Could you check a few things on this drawing? It's one solid part, dimensions in mm from its lowest x, y, z. A direction names the side the tool comes from. Give positions to 0.01 mm unless a question says otherwise; leave off trailing zeros. Order: outer loops, then holes, each group sorted by start corner. A loop starts at its lowest first (then second) coordinate and runs counter-clockwise, first axis right, second up.
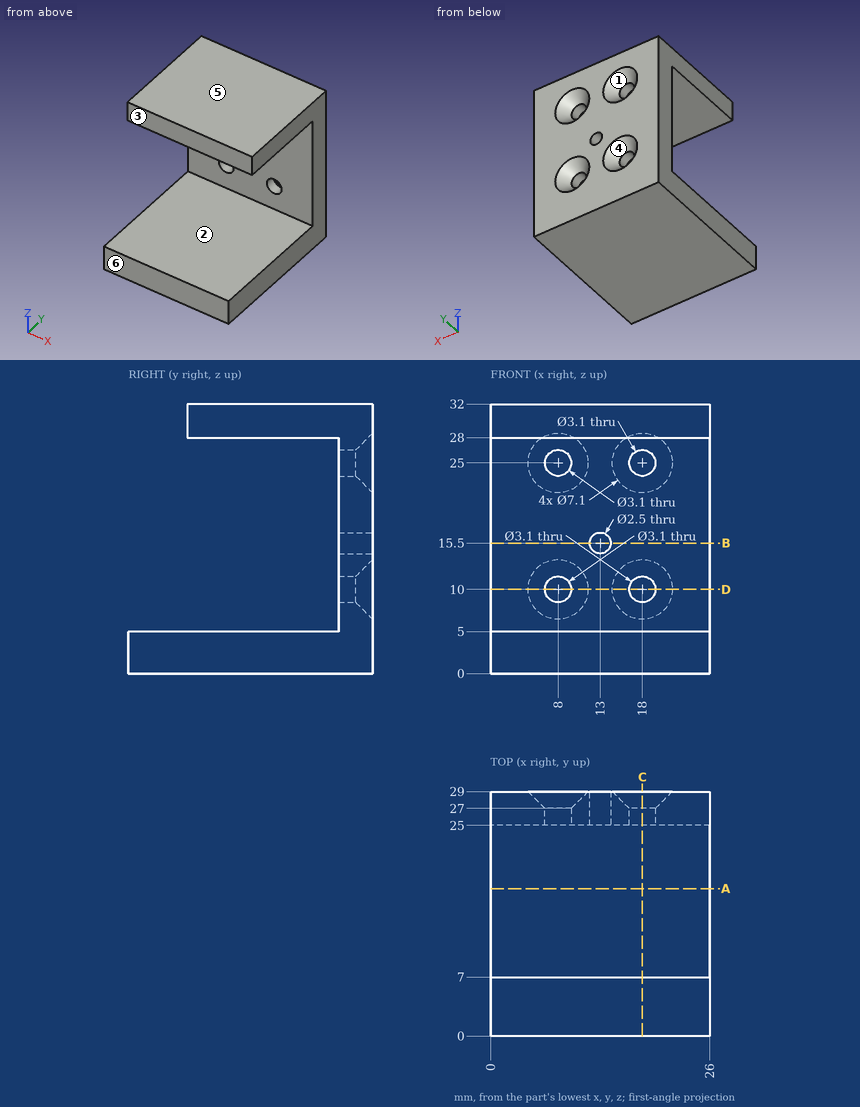
Item 1: For pin 1 (5 mm diameter, centred on x = 8, z = 25, fed in from -Y); pin 2 (4 mm diameter, centred on x = 8, z = 10, fed in from +Y); pin 3 (3 mm diameter, centred on x = 10, z = 31, fed in from -Y), each with a flat end and sliding along its axis, tell me the tip position at first contact or that it passes through.
Findings:
pin 1: stops at y = 25
pin 2: stops at y = 27.45
pin 3: stops at y = 7
Item 2: Imagine slicing it at A-A on y = 17.5. List the corners of the cut face in (x, z) for me.
Findings:
outline: (0, 0) - (26, 0) - (26, 5) - (0, 5) - close; (0, 28) - (26, 28) - (26, 32) - (0, 32) - close
Item 3: For the marked faces 1, 2 and 3, which set-ups out of +Z, -Z, +X, -X, +Y, -Y let a thin tool reach every point of the face, with its end or its side?
Findings:
face 1: +Y
face 2: +X, -X, -Y
face 3: +Z, +X, -X, -Y
Item 4: Imagine slicing it at D-D on z = 10. List the corners of the cut face in (x, y) for me, then the cut area to 3 significant figures.
Findings:
outline: (0, 25) - (6.45, 25) - (6.45, 27) - (4.45, 29) - (0, 29) - close; (9.55, 25) - (16.45, 25) - (16.45, 27) - (14.45, 29) - (11.55, 29) - (9.55, 27) - close; (19.55, 25) - (26, 25) - (26, 29) - (21.55, 29) - (19.55, 27) - close
area: 71.2 mm2
Item 5: Imagine slicing it at C-C on x = 18. List the corners of the cut face in (y, z) for me, then the cut area to 3 significant figures.
Findings:
outline: (0, 0) - (29, 0) - (29, 6.45) - (27, 8.45) - (25, 8.45) - (25, 5) - (0, 5) - close; (7, 28) - (25, 28) - (25, 26.55) - (27, 26.55) - (29, 28.55) - (29, 32) - (7, 32) - close; (25, 11.55) - (27, 11.55) - (29, 13.55) - (29, 21.45) - (27, 23.45) - (25, 23.45) - close
area: 292 mm2
Item 6: Imagine slicing it at B-B on z = 15.5. List the corners of the cut face in (x, y) for me.
Findings:
outline: (0, 25) - (11.75, 25) - (11.75, 29) - (0, 29) - close; (14.25, 25) - (26, 25) - (26, 29) - (14.25, 29) - close
Item 7: We'd pull the mould along Z, two halves only. Please class the marked faces 4, 5 and 6: +Z half, -Z half, draft (parallel to the pull), parting line (faces both ways), or undercut.
Findings:
face 4: undercut
face 5: +Z half
face 6: draft
Item 8: Please list where these lines run through material, in increasing order: line 1 along Z through (x, y) = (18, 25.75); line 2 along Z through (x, y) = (20.5, 17); line 3 along X through (y, z) = (26.4, 25).
Findings:
line 1: z = 0 to 8.45, 11.55 to 23.45, 26.55 to 32
line 2: z = 0 to 5, 28 to 32
line 3: x = 0 to 6.45, 9.55 to 16.45, 19.55 to 26
